from build123d import *

# Parameters (mm, degrees)
F1_DEPTH  = 101.6
F3_DEPTH  = 2.54
F5_DEPTH  = 114.3
F6_W      = 50.8
F6_H      = 63.5
F6_W_2    = 38.1
F6_H_2    = 50.8
F7_DEPTH  = 2.54
F8_W      = 63.5
F8_H      = 19.05
F9_DEPTH  = 19.05
F10_W     = 13.716
F10_H     = 58.42
F11_DEPTH = 15.24


with BuildPart() as f1:
    # F0 (on Front) → F1 (new body, symmetric)
    with BuildSketch(Plane.XZ):
        Polygon((-76.2, 167.667356), (-76.2, 0), (76.2, 0), (76.2, 167.667356), (0, 203.2), align=None)
    extrude(amount=F1_DEPTH, both=True)

    # F2 (on face) → F3 (join)
    with BuildSketch(Plane.XZ.offset(101.6)):
        Polygon((-37.118237, 0), (-37.118237, 152.4), (39.081763, 152.4), (39.081763, 0), (45.431763, 0), (45.431763, 158.75), (-43.468237, 158.75), (-43.468237, 0), align=None)
    extrude(amount=F3_DEPTH)

    # F4 (on Front) → F5 (join, symmetric)
    with BuildSketch(Plane.XZ):
        Polygon((97.933626, 157.5328), (0, 203.2), (-97.933626, 157.5328), (-95.25, 151.777746), (0, 196.19355), (95.25, 151.777746), align=None)
    extrude(amount=F5_DEPTH, both=True)

    # F6 (on face) → F7 (join)
    with BuildSketch(Plane(origin=(-76.2, 0, 0), x_dir=(0, -1, 0), z_dir=(-1, 0, 0))):
        with Locations((-50.8, 101.6)):
            Rectangle(F6_W, F6_H)
        with Locations((-50.8, 101.6)):
            Rectangle(F6_W_2, F6_H_2, mode=Mode.SUBTRACT)
        with Locations((50.8, 101.6)):
            Rectangle(F6_W, F6_H)
        with Locations((50.8, 101.6)):
            Rectangle(F6_W_2, F6_H_2, mode=Mode.SUBTRACT)
    extrude(amount=F7_DEPTH)

    # F8 (on face) → F9 (join)
    with BuildSketch(Plane(origin=(-76.2, 0, 0), x_dir=(0, -1, 0), z_dir=(-1, 0, 0))):
        with Locations((-50.8, 60.325)):
            Rectangle(F8_W, F8_H)
        with Locations((50.8, 60.325)):
            Rectangle(F8_W, F8_H)
    extrude(amount=F9_DEPTH)

    # F10 (on face) → F11 (cut)
    with BuildSketch(Plane.XY.offset(69.85)):
        with Locations((-85.852, 50.8)):
            Rectangle(F10_W, F10_H)
        with Locations((-85.852, -50.8)):
            Rectangle(F10_W, F10_H)
    extrude(amount=-F11_DEPTH, mode=Mode.SUBTRACT)


solid = f1.part
Work out the finished part from the listing and answer in its coordinate system (mm). A direction names the side the tool comes from. Give positions to 0.01 mm unless a question says otherwise; leave off trailing zeros. Loops run counter-clockwise (first coordinate to the right, second up) from the corner with the lowest first, then second, coordinate; pieces in that order, holes last. Notation, with made-up numbers: (72, 71) - (114, 71) arc R13 cw to (114, 81) - close; hole circle Ø5 at (-31, 61.25). An arc over 180 degrees is marked (long way). Answer in a Markdown table with one row per item.
(1) Section A-A (z = 145) is taken. Give the vertices of the cut face in (x, y).
Results list:
| item | result |
|---|---|
| outline | (-76.2, -101.6) - (-43.47, -101.6) - (-43.47, -104.14) - (-37.12, -104.14) - (-37.12, -101.6) - (39.08, -101.6) - (39.08, -104.14) - (45.43, -104.14) - (45.43, -101.6) - (76.2, -101.6) - (76.2, 101.6) - (-76.2, 101.6) - close |
(2) Section B-B (x = 60.5) is taken. Give the vertices of the cut face in (y, z).
Results list:
| item | result |
|---|---|
| outline | (-114.3, 167.98) - (-101.6, 167.98) - (-101.6, 0) - (101.6, 0) - (101.6, 167.98) - (114.3, 167.98) - (114.3, 174.99) - (-114.3, 174.99) - close |
(3) Section C-C (y = 63) is taken. Give the vertices of the cut face in (x, z).
Results list:
| item | result |
|---|---|
| outline | (-97.93, 157.53) - (-95.25, 151.78) - (-76.2, 160.66) - (-76.2, 133.35) - (-78.74, 133.35) - (-78.74, 127) - (-76.2, 127) - (-76.2, 76.2) - (-78.74, 76.2) - (-78.74, 69.85) - (-78.99, 69.85) - (-78.99, 54.61) - (-92.71, 54.61) - (-92.71, 69.85) - (-95.25, 69.85) - (-95.25, 50.8) - (-76.2, 50.8) - (-76.2, 0) - (76.2, 0) - (76.2, 160.66) - (95.25, 151.78) - (97.93, 157.53) - (0, 203.2) - close |
(4) For a pull along Z with two mould halves and no side action, classify faces 6 (the face through (-86, 51, 50.8)), 7 (the face through (-95.25, -50, 60)), 8 (the face through (-78.994, 50, 62)) as pulls with the +Z half, pulls with the -Z half, needs draft (parallel to the pull), parting line crosses it, or undercut.
Results list:
| item | result |
|---|---|
| face 6 | pulls with the -Z half |
| face 7 | needs draft |
| face 8 | undercut |
(5) A tool of negligible diameter and unlimited length cuts with its end or side. For faces 1 (the face through (-76.2, -51, 102)), 2 (the face through (-78.74, -73, 102)), 3 (the face through (-39, -104.14, 92)), 4 (the face through (-86, 80.01, 62)), 5 (the face through (-1, -3, 0)), from which of +Z, -Z, +X, -X, +Y, -Y can it reach the whole face along a straight path? Write none if from no direction.
Results list:
| item | result |
|---|---|
| face 1 | -X |
| face 2 | -X, +Y, -Y |
| face 3 | -Z, -Y |
| face 4 | none |
| face 5 | -Z, +X, -X, +Y, -Y |
(6) Consider L1, parallel to X at y = 73, z = 76; L2, parallel to X at y = -18.5, z = 73.5; L3, parallel to Y at x = -35, z = 66.5. Determine where each line is inside the solid, lowest interval first. Write a range as [from, to].
Results list:
| item | result |
|---|---|
| L1 | x = [-78.74, 76.2] |
| L2 | x = [-76.2, 76.2] |
| L3 | y = [-101.6, 101.6] |
(7) Flat-ended cylindrical pins translate along their axes: pin 1 Ø1.5 at (x, y) = (-32.5, -31) entering from +Z; pin 2 Ø5.5 at (y, z) = (66, 57) entering from -X; pin 3 Ø1 at (y, z) = (-90, 57) entering from -X. Find the tip coordinate at first contact, or state that the pin passes through.
Results list:
| item | result |
|---|---|
| pin 1 | stops at z = 188.39 |
| pin 2 | stops at x = -95.25 |
| pin 3 | stops at x = -76.2 |
(8) Section D-D (z = 112) is taken. Give the vertices of the cut face in (x, y), and give its area (3 significant figures).
Results list:
| item | result |
|---|---|
| outline | (-78.74, -76.2) - (-76.2, -76.2) - (-76.2, -101.6) - (-43.47, -101.6) - (-43.47, -104.14) - (-37.12, -104.14) - (-37.12, -101.6) - (39.08, -101.6) - (39.08, -104.14) - (45.43, -104.14) - (45.43, -101.6) - (76.2, -101.6) - (76.2, 101.6) - (-76.2, 101.6) - (-76.2, 76.2) - (-78.74, 76.2) - (-78.74, 69.85) - (-76.2, 69.85) - (-76.2, 31.75) - (-78.74, 31.75) - (-78.74, 25.4) - (-76.2, 25.4) - (-76.2, -25.4) - (-78.74, -25.4) - (-78.74, -31.75) - (-76.2, -31.75) - (-76.2, -69.85) - (-78.74, -69.85) - close |
| area | 31,100 mm² |
